from build123d import *

# Parameters (mm, degrees)
BOSS_EXTRUDE1_DEPTH = 12.7
CUT_EXTRUDE1_REACH  = 58.199
SKETCH2_R           = 1.5875


with BuildPart() as part:
    # Sketch1 → Boss-Extrude1 (new body)
    with BuildSketch(Plane.XY):
        Polygon((25.4, 0), (49.268192568, 23.868192568), (49.268192568, 26.408192568), (25.4, 17.720880927), (25.4, 5.08), (22.86, 2.54), (0, 2.54), (0, 0), align=None)
    boss_extrude1 = extrude(amount=BOSS_EXTRUDE1_DEPTH)

    # Mirror1: Boss-Extrude1 across plane
    add(boss_extrude1.mirror(Plane(origin=(0, 0, 12.7), x_dir=(0, 0, 1), z_dir=(1, 0, 0))))

    # Sketch2 → Cut-Extrude1 (cut, up to next)
    with BuildSketch(Plane(origin=(0, 2.54, 0), x_dir=(1, 0, 0), z_dir=(0, 1, 0)), mode=Mode.PRIVATE) as cut_extrude1_sk1:
        with BuildLine():
            ThreePointArc((-12.550350762, -6.35), (-14.137850762, -4.7625), (-15.725350762, -6.35))
            Line((-15.725350762, -6.35), (-12.550350762, -6.35))
        make_face()
    cut_extrude1_tool1 = extrude(cut_extrude1_sk1.sketch, amount=-CUT_EXTRUDE1_REACH, mode=Mode.PRIVATE) & part.part
    # Sketch2 → Cut-Extrude1 (cut, up to next)
    with BuildSketch(Plane(origin=(0, 2.54, 0), x_dir=(1, 0, 0), z_dir=(0, 1, 0)), mode=Mode.PRIVATE) as cut_extrude1_sk2:
        with Locations(Location((14.137850762, -6.35, 0), (0, 0, 270))):
            Circle(SKETCH2_R)
    cut_extrude1_tool2 = extrude(cut_extrude1_sk2.sketch, amount=-CUT_EXTRUDE1_REACH, mode=Mode.PRIVATE) & part.part
    add(cut_extrude1_tool1.solids().sort_by_distance((-14.137851, 2.54, 5.676244))[0], mode=Mode.SUBTRACT)
    add(cut_extrude1_tool2.solids().sort_by_distance((14.137851, 2.54, 6.35))[0], mode=Mode.SUBTRACT)


solid = part.part
Source: CAD feature listing. Evaluate the final solid. Frame: model axes, mm. A direction names the side the tool comes from. Round coordinates to 2 decimals unless told otherwise and drop trailing zeros. Loops run counter-clockwise (first coordinate to the right, second up) from the corner with the lowest first, then second, coordinate; pieces in that order, holes last. Notation, with made-up numbers: (23.5, 49.25) - (45.5, 49.25) arc R28 ccw to (45.5, 82.25) - close; hole circle Ø3 at (-13.75, -25). An arc over 180 degrees is marked (long way). Write item = value, one per line. Start each with the question number.
Item 1: Section query C-C on y = 4.25. Output: boundary loops of the cut face in (x, z), plus the area to 3 significant figures.
Item 2: Section query D-D on x = 17. Output: boundary loops of the cut face in (y, z), plus the area to 3 significant figures.
Item 3: First-contact query: pin 1 Ø1.5 at (x, z) = (21, 8) entering from +Y; pin 2 Ø3 at (x, z) = (28.5, 10.5) entering from -Y; pin 3 Ø2 at (y, z) = (18.5, 7) entering from +X; pin 4 Ø3 at (x, y) = (-14.5, 2) entering from -Z. Flat tips, straight axial feed; report the tip coordinate or a pass-through.
Item 4: Mould query, pull axis X, two halves, no side actions, for faces 4 (the face through (0, 2, 0)), 5 (the face through (-37.2, 11.8, 6.3)), 6 (the face through (-24.15, 3.83, 6.26)). Classes: released by +X, released by -X, zero draft, split by the parting line, or undercut.
Item 5: Section query A-A on y = 12.75. Output: boundary loops of the cut face in (x, z), plus the area to 3 significant figures.
Item 6: Section query B-B on z = 10.5. Output: boundary loops of the cut face in (x, y).
Item 7: Reachability of faces 1 (the face through (25.4, 11, 6)), 2 (the face through (-14, 1, 6.35)), 3 (the face through (-49.268, 25, 6)) from +Z, -Z, +X, -X, +Y, -Y: full face, straight path, thin tool, end or side. Return the list, or none.
Item 8: Material intervals for line 1 (Y direction, x = 11, z = 8); line 2 (X direction, y = 9, z = 2.5); line 3 (Z direction, x = 14.5, y = 2), sorted ascending.
Results list:
q1.outline = (-29.65, 0) - (-24.57, 0) - (-24.57, 12.7) - (-29.65, 12.7) - close; (24.57, 0) - (29.65, 0) - (29.65, 12.7) - (24.57, 12.7) - close
q1.area = 129 mm²
q2.outline = (0, 0) - (2.54, 0) - (2.54, 12.7) - (0, 12.7) - close
q2.area = 32.3 mm²
q3.pin_1 = 2.54
q3.pin_2 = 1.6
q3.pin_3 = 44.9
q3.pin_4 = 0
q4.face_4 = zero draft
q4.face_5 = released by -X
q4.face_6 = undercut
q5.outline = (-38.15, 0) - (-25.4, 0) - (-25.4, 12.7) - (-38.15, 12.7) - close; (25.4, 0) - (38.15, 0) - (38.15, 12.7) - (25.4, 12.7) - close
q5.area = 324 mm²
q6.outline = (-49.27, 23.87) - (-25.4, 0) - (25.4, 0) - (49.27, 23.87) - (49.27, 26.41) - (25.4, 17.72) - (25.4, 5.08) - (22.86, 2.54) - (-22.86, 2.54) - (-25.4, 5.08) - (-25.4, 17.72) - (-49.27, 26.41) - close
q7.face_1 = +Z, -Z, +Y
q7.face_2 = +Y, -Y
q7.face_3 = +Z, -Z, -X, +Y, -Y
q8.line_1 = 0 to 2.54
q8.line_2 = -34.4 to -25.4, 25.4 to 34.4
q8.line_3 = 0 to 4.8, 7.9 to 12.7
